```python
from build123d import *

# Parameters (mm, degrees)
SKETCH1_R           = 40
BOSS_EXTRUDE1_DEPTH = 13
CUT_EXTRUDE1_DEPTH  = 8
SKETCH2_4_R         = 1.4
CUT_EXTRUDE2_DEPTH  = 5
SKETCH3_W           = 14
SKETCH3_H           = 28
CUT_EXTRUDE6_DEPTH  = 10
SKETCH5_R           = 45
BOSS_EXTRUDE2_DEPTH = 4
SKETCH6_R           = 1.4
CUT_EXTRUDE8_DEPTH  = 4
SKETCH6_3_R         = 1.4
CUT_EXTRUDE9_DEPTH  = 4
SKETCH7_W           = 14
SKETCH7_H           = 14
CUT_EXTRUDE10_DEPTH = 17


with BuildPart() as part:
    # Sketch1 → Boss-Extrude1 (new body)
    with BuildSketch(Plane.XY):
        with Locations(Location((0, 0, 0), (0, 0, 180))):
            Circle(SKETCH1_R)
    extrude(amount=BOSS_EXTRUDE1_DEPTH)

    # Sketch2 → Cut-Extrude1 (cut)
    with BuildSketch(Plane.XY.offset(13)):
        Polygon((-40, 12), (-40, -12), (-20, -12), (-20, -17), (-9, -17), (-9, -3.5), (-1, -3.5), (-1, 3.5), (-9, 3.5), (-9, 17), (-20, 17), (-20, 12), align=None)
        Polygon((1, 3.5), (1, -3.5), (9, -3.5), (9, -17), (20, -17), (20, -12), (40, -12), (40, 12), (20, 12), (20, 17), (9, 17), (9, 3.5), align=None)
    extrude(amount=-CUT_EXTRUDE1_DEPTH, mode=Mode.SUBTRACT)

    # Sketch2_4 → Cut-Extrude2 (cut)
    with BuildSketch(Plane.XY.offset(13)):
        with Locations((20, 20)):
            Circle(SKETCH2_4_R)
        with Locations((-20, -20)):
            Circle(SKETCH2_4_R)
        with Locations((20, -20)):
            Circle(SKETCH2_4_R)
        with Locations((-20, 20)):
            Circle(SKETCH2_4_R)
    extrude(amount=-CUT_EXTRUDE2_DEPTH, mode=Mode.SUBTRACT)

    # Sketch3 → Cut-Extrude6 (cut)
    with BuildSketch(Plane.XY.offset(13)):
        with Locations((0, -19)):
            Rectangle(SKETCH3_W, SKETCH3_H)
        with Locations((0, 19)):
            Rectangle(SKETCH3_W, SKETCH3_H)
    extrude(amount=-CUT_EXTRUDE6_DEPTH, mode=Mode.SUBTRACT)

    # Sketch5 → Boss-Extrude2 (add)
    with BuildSketch(Plane(origin=(0, 0, 0), x_dir=(-1, 0, 0), z_dir=(0, 0, -1))):
        Circle(SKETCH5_R)
    extrude(amount=BOSS_EXTRUDE2_DEPTH)

    # Sketch6 → Cut-Extrude8 (cut)
    with BuildSketch(Plane(origin=(0, 0, 0), x_dir=(-1, 0, 0), z_dir=(0, 0, -1))):
        with Locations((0, 42.5)):
            Circle(SKETCH6_R)
        with Locations((30.0520382, 30.0520382)):
            Circle(SKETCH6_R)
        with Locations((42.5, 0)):
            Circle(SKETCH6_R)
        with Locations((30.0520382, -30.0520382)):
            Circle(SKETCH6_R)
        with Locations((0, -42.5)):
            Circle(SKETCH6_R)
        with Locations((-30.0520382, -30.0520382)):
            Circle(SKETCH6_R)
        with Locations((-42.5, 0)):
            Circle(SKETCH6_R)
        with Locations((-30.0520382, 30.0520382)):
            Circle(SKETCH6_R)
    extrude(amount=CUT_EXTRUDE8_DEPTH, mode=Mode.SUBTRACT)

    # Sketch6_3 → Cut-Extrude9 (cut)
    with BuildSketch(Plane(origin=(0, 0, 0), x_dir=(-1, 0, 0), z_dir=(0, 0, -1))):
        with Locations((0, 32.5)):
            Circle(SKETCH6_3_R)
        with Locations((22.980970389, 22.980970389)):
            Circle(SKETCH6_3_R)
        with Locations((32.5, 0)):
            Circle(SKETCH6_3_R)
        with Locations((22.980970389, -22.980970389)):
            Circle(SKETCH6_3_R)
        with Locations((0, -32.5)):
            Circle(SKETCH6_3_R)
        with Locations((-22.980970389, -22.980970389)):
            Circle(SKETCH6_3_R)
        with Locations((-32.5, 0)):
            Circle(SKETCH6_3_R)
        with Locations((-22.980970389, 22.980970389)):
            Circle(SKETCH6_3_R)
    extrude(amount=CUT_EXTRUDE9_DEPTH, mode=Mode.SUBTRACT)

    # Sketch7 → Cut-Extrude10 (cut)
    with BuildSketch(Plane.XY.offset(13)):
        with Locations((0, 12)):
            Rectangle(SKETCH7_W, SKETCH7_H)
        with Locations((0, -12)):
            Rectangle(SKETCH7_W, SKETCH7_H)
    extrude(amount=-CUT_EXTRUDE10_DEPTH, mode=Mode.SUBTRACT)


solid = part.part
```
Source: CAD feature listing. Evaluate the final solid. Frame: model axes, mm. A direction names the side the tool comes from. Round coordinates to 2 decimals unless told otherwise and drop trailing zeros. Loops run counter-clockwise (first coordinate to the right, second up) from the corner with the lowest first, then second, coordinate; pieces in that order, holes last. Notation, with made-up numbers: (78, 0.25) - (116, 0.25) arc R31 cw to (116, 33.25) - close; hole circle Ø7 at (-11, 55.25). An arc over 180 degrees is marked (long way). Use CSV: the item, a comma, the result in double quotes.
Q1. Reachability of faces 1 (the flat face through (-7, 16, 7)), 2 (the flat face through (-23, 23, 0)), 3 (the flat face through (29, -12, 9)) from +Z, -Z, +X, -X, +Y, -Y: full face, straight path, thin tool, end or side. Return the list, or none.
Reported:
face 1,"+Z"
face 2,"-Z"
face 3,"+Z, +X"
Q2. Section query B-B, the plane y = -8. Output: boundary loops of the cut face in (x, z).
Reported:
outline,"(-44.28, -4) - (-7, -4) - (-7, 13) - (-9, 13) - (-9, 5) - (-39.19, 5) - (-39.19, 0) - (-44.28, 0) - close; (7, -4) - (44.28, -4) - (44.28, 0) - (39.19, 0) - (39.19, 5) - (9, 5) - (9, 13) - (7, 13) - close"
Q3. Section query C-C, the plane y = 36. Output: boundary loops of the cut face in (x, z), then the cut area to 3 significant figures.
Reported:
outline,"(-27, -4) - (27, -4) - (27, 0) - (17.44, 0) - (17.44, 13) - (-17.44, 13) - (-17.44, 0) - (-27, 0) - close"
area,"669 mm^2"
Q4. Ray query, line 1 along X through (y, z) = (-24, -1); line 2 along X through (y, z) = (-13, 5.5); line 3 along Z through (x, y) = (36.5, 11). Return the intervals inside material, ascending.
Reported:
line 1,"-38.07 to -23.94, -22.02 to 22.02, 23.94 to 38.07"
line 2,"-37.83 to -20, -9 to -7, 7 to 9, 20 to 37.83"
line 3,"-4 to 5"
Q5. Section query A-A, the plane x = -42.5. Output: boundary loops of the cut face in (y, z).
Reported:
outline,"(-14.79, -4) - (-1.4, -4) - (-1.4, 0) - (-14.79, 0) - close; (1.4, -4) - (14.79, -4) - (14.79, 0) - (1.4, 0) - close"
Q6. Section query D-D, the plane z = 9.5. Give the number of separate pieces and of enclosed holes in the cut face, then the cut area to 3 significant figures.
Reported:
separate pieces,"1"
enclosed holes,"6"
area,"2,430 mm^2"
Q7. Pin query (flat end, axial travel): pin 1 Ø4 at (y, z) = (14.5, 8) entering from +X; pin 2 Ø5 at (x, y) = (-16.5, 3) entering from +Z; pin 3 Ø5.5 at (x, z) = (-3, -1) entering from -Y. Return the tip coordinate at first contact, or that it passes through.
Reported:
pin 1,"x = 38"
pin 2,"z = 5"
pin 3,"y = -45"
